```python
from build123d import *

# Parameters (mm, degrees)
SKETCH1_W           = 130
SKETCH1_H           = 67.5
SKETCH1_R           = 1.7
BOSS_EXTRUDE1_DEPTH = 1.5
SKETCH2_R           = 5
BOSS_EXTRUDE2_DEPTH = 8
SKETCH3_R           = 5
BOSS_EXTRUDE3_DEPTH = 5
SKETCH4_R           = 10
BOSS_EXTRUDE4_DEPTH = 15
SKETCH5_W           = 8
SKETCH5_H           = 8
BOSS_EXTRUDE5_DEPTH = 3
SKETCH6_R           = 2.5
BOSS_EXTRUDE6_DEPTH = 10
SKETCH7_W           = 50
SKETCH7_H           = 7.5
BOSS_EXTRUDE7_DEPTH = 5
SKETCH8_W           = 52
SKETCH8_H           = 1.5
BOSS_EXTRUDE8_DEPTH = 1.5


with BuildPart() as part:
    # Sketch1 → Boss-Extrude1 (new body)
    with BuildSketch(Plane.XY):
        with Locations((62, 30.75)):
            Rectangle(SKETCH1_W, SKETCH1_H)
        Circle(SKETCH1_R, mode=Mode.SUBTRACT)
        with Locations((0, 61.5)):
            Circle(SKETCH1_R, mode=Mode.SUBTRACT)
        with Locations((124, 61.5)):
            Circle(SKETCH1_R, mode=Mode.SUBTRACT)
        with Locations((124, 0)):
            Circle(SKETCH1_R, mode=Mode.SUBTRACT)
    extrude(amount=BOSS_EXTRUDE1_DEPTH)

    # Sketch2 → Boss-Extrude2 (add)
    with BuildSketch(Plane.XY.offset(1.5)):
        with Locations(Location((114.5, 56, 0), (0, 0, 180))):
            Circle(SKETCH2_R)
    extrude(amount=BOSS_EXTRUDE2_DEPTH)

    # Sketch3 → Boss-Extrude3 (add)
    with BuildSketch(Plane.XY.offset(1.5)):
        with Locations(Location((114.5, 34, 0), (0, 0, 180))):
            Circle(SKETCH3_R)
    extrude(amount=BOSS_EXTRUDE3_DEPTH)

    # Sketch4 → Boss-Extrude4 (add)
    with BuildSketch(Plane.XY.offset(6.5)):
        with Locations((114.5, 34)):
            Circle(SKETCH4_R)
    extrude(amount=BOSS_EXTRUDE4_DEPTH)

    # Sketch5 → Boss-Extrude5 (add)
    with BuildSketch(Plane.XY.offset(1.5)):
        with Locations((114.5, 9.5)):
            Rectangle(SKETCH5_W, SKETCH5_H)
    extrude(amount=BOSS_EXTRUDE5_DEPTH)

    # Sketch6 → Boss-Extrude6 (add)
    with BuildSketch(Plane.XY.offset(4.5)):
        with Locations((114.5, 9.5)):
            Circle(SKETCH6_R)
    extrude(amount=BOSS_EXTRUDE6_DEPTH)

    # Sketch7 → Boss-Extrude7 (add)
    with BuildSketch(Plane(origin=(0, 0, 0), x_dir=(-1, 0, 0), z_dir=(0, 0, -1))):
        with Locations((-55, 32.75)):
            Rectangle(SKETCH7_W, SKETCH7_H)
    extrude(amount=BOSS_EXTRUDE7_DEPTH)

    # Sketch8 → Boss-Extrude8 (add)
    with BuildSketch(Plane(origin=(0, 0, 0), x_dir=(-1, 0, 0), z_dir=(0, 0, -1))):
        with Locations((-44.5, -0.25)):
            Rectangle(SKETCH8_W, SKETCH8_H)
    extrude(amount=BOSS_EXTRUDE8_DEPTH)


solid = part.part
```
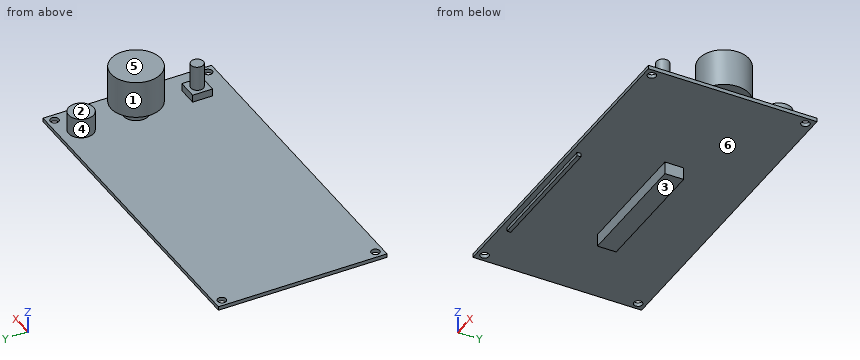
Could you check a few things on this model? Use its own coordinates, in mm. Face numbers are marked on the shaded views. A direction names the side the tool comes from. Round coordinates to 2 decimals unless told otherwise and drop trailing zeros. Loops run counter-clockwise (first coordinate to the right, second up) from the corner with the lowest first, then second, coordinate; pieces in that order, holes last. Notation, with made-up numbers: M 16.5,-35 L 67.5,-35 A16 cw 67.5,-8 Z; hole C 77.5,60 d4. An arc over 180 degrees is marked long. Put each result on its own line as item: value.
Q1. Imagine slicing it at B-B (y = 34). Write out the boundary of the cut face in (x, z).
Check result:
outline: M -3,0 L 30,0 L 30,-5 L 80,-5 L 80,0 L 127,0 L 127,1.5 L 119.5,1.5 L 119.5,6.5 L 124.5,6.5 L 124.5,21.5 L 104.5,21.5 L 104.5,6.5 L 109.5,6.5 L 109.5,1.5 L -3,1.5 Z
Q2. Imagine slicing it at C-C (x = 66.5). Write out the boundary of the cut face in (y, z).
Check result:
outline: M -3,0 L -1,0 L -1,-1.5 L 0.5,-1.5 L 0.5,0 L 29,0 L 29,-5 L 36.5,-5 L 36.5,0 L 64.5,0 L 64.5,1.5 L -3,1.5 Z
Q3. For pin 1 (2.5 mm diameter, centred on y = 34.5, z = -3, fed in from -X); pin 2 (4.5 mm diameter, centred on x = 124, y = 61.5, fed in from -Z); pin 3 (2 mm diameter, centred on y = 28, z = 6, fed in from -X); pin 4 (2 mm diameter, centred on x = 0, y = 0, fed in from -Z), each with a flat end and sliding along its axis, tell me the tip position at first contact or that it passes through.
Check result:
pin 1: x = 30
pin 2: z = 0
pin 3: x = 105.92
pin 4: through
Q4. Imagine slicing it at D-D (z = 11.25). Write out the boundary of the cut face in (x, y).
Check result:
outline: C 114.5,34 d20; C 114.5,9.5 d5
Q5. On a 3-axis mill with a long thin cutter (end or side, diameter ignored), from which of +Z, -Z, +X, -X, +Y, -Y can I reach the whole of each face in a straight line? I mean the marked faces 1, 2 and 3. Say none if no direction works.
Check result:
face 1: +Z
face 2: +Z, +X, -X, +Y
face 3: -Z, +X, -X, +Y, -Y
Q6. Imagine slicing it at A-A (x = 0). Write out the boundary of the cut face in (y, z).
Check result:
outline: M -3,0 L -1.7,0 L -1.7,1.5 L -3,1.5 Z; M 1.7,0 L 59.8,0 L 59.8,1.5 L 1.7,1.5 Z; M 63.2,0 L 64.5,0 L 64.5,1.5 L 63.2,1.5 Z
Q7. Thinking about a two-plate mould opening in Y: for the marked faces 4, 5 and 6, which applies, released by +Y, released by -Y, zero draft, split by the parting line, or undercut?
Check result:
face 4: undercut
face 5: zero draft
face 6: undercut
Q8. I need wall thicknesses on probe 1 along Y at (x, z) = (0, 1); probe 2 along Y at (x, z) = (113.5, 2.5); probe 3 along Z at (x, y) = (114, 42). Which ranges of each line are inside material? Lowest first, please.
Check result:
probe 1: -3 to -1.7, 1.7 to 59.8, 63.2 to 64.5
probe 2: 5.5 to 13.5, 29.1 to 38.9, 51.1 to 60.9
probe 3: 0 to 1.5, 6.5 to 21.5
